```python
from build123d import *

# Parameters (mm, degrees)
EXTRUDE_THIN1_DEPTH = 3.175


with BuildPart() as part:
    # Sketch1 → Extrude-Thin1 (new, symmetric)
    with BuildSketch(Plane(origin=(0, 0, 0), x_dir=(0, 0, -1), z_dir=(1, 0, 0))):
        with BuildLine():
            ThreePointArc((-19.05, 0.3048), (-14.081230666, 0.814453346), (-9.525000281, 2.861201965))
            ThreePointArc((-9.525000281, 2.861201965), (0, 5.715), (9.525000281, 2.861201965))
            ThreePointArc((9.525000281, 2.861201965), (14.081230666, 0.814453346), (19.05, 0.3048))
            Line((19.05, 0.3048), (19.067602036, 0.000508679))
            ThreePointArc((19.067602036, 0.000508679), (14.002221921, 0.520071522), (9.357401999, 2.606616309))
            ThreePointArc((9.357401999, 2.606616309), (0, 5.4102), (-9.357401999, 2.606616309))
            ThreePointArc((-9.357401999, 2.606616309), (-14.002221921, 0.520071522), (-19.067602036, 0.000508679))
            Line((-19.067602036, 0.000508679), (-19.05, 0.3048))
        make_face()
    extrude(amount=EXTRUDE_THIN1_DEPTH, both=True)


solid = part.part
```
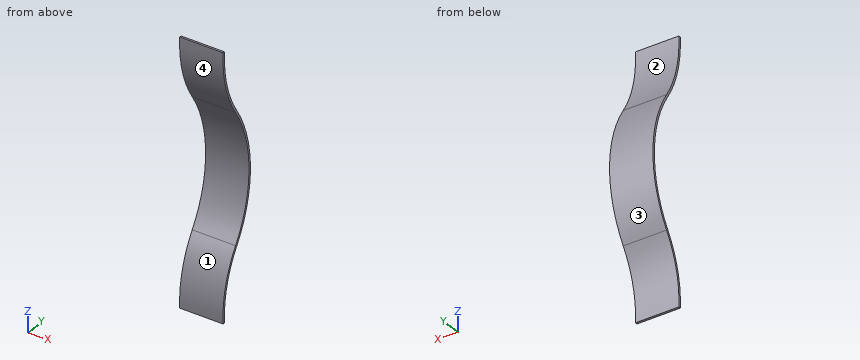
Part model, mm, in its own coordinate system. Face numbers are marked on the shaded views. A direction names the side the tool comes from. Coordinates: 2 decimals unless noted, no trailing zeros. Write each loop counter-clockwise with the first axis right and the second up, starting at its lowest first coordinate (ties: lowest second). Pieces come first, ordered by that corner, then holes.
Item 1: Pin check, flat tip, straight feed: pin 1 (1 mm diameter, centred on y = 2.5, z = 4, fed in from -X). Stop position of the tip, or through.
Item 2: Probe line 1 (Z direction, x = -1.25, y = 1.8); line 2 (Z direction, x = -0.25, y = 3.5); line 3 (Y direction, x = 1.5, z = 0) (3 decimals). List the from-to ranges inside material, lowest first.
Item 3: Slice it at C-C (y = 3.95). Write the cut outline in (x, z) (3 decimals), and give its area (3 significant figures).
Item 4: Which spindle directions (+Z, -Z, +X, -X, +Y, -Y) get a long thin tool onto all of the face, cutting with end or side? Do the marked faces 1 and 2. Say none if no direction does.
Item 5: Mould opens along Z. For the marked faces 3 and 4 say: released by +Z, released by -Z, zero draft, split by the parting line, or undercut.
Item 6: Slice it at D-D (z = -2). Write the cut outline in (x, y) (3 decimals).
Item 7: Slice it at A-A (y = 1.25). Write the cut outline in (x, z) (3 decimals).
Results found:
1. pin 1: passes through
2. line 1: z = -11.41 to -10.73, 10.73 to 11.41
2. line 2: z = -8.48 to -7.83, 7.83 to 8.48
2. line 3: y = 5.41 to 5.715
3. outline: (-3.175, -7.618) - (3.175, -7.618) - (3.175, -6.897) - (-3.175, -6.897) - close; (-3.175, 6.897) - (3.175, 6.897) - (3.175, 7.618) - (-3.175, 7.618) - close
3. area: 9.16 mm2
4. face 1: +X, -X, -Y
4. face 2: +X, -X, +Y
5. face 3: split by the parting line
5. face 4: undercut
6. outline: (-3.175, 5.292) - (3.175, 5.292) - (3.175, 5.599) - (-3.175, 5.599) - close
7. outline: (-3.175, -12.712) - (3.175, -12.712) - (3.175, -11.887) - (-3.175, -11.887) - close; (-3.175, 11.887) - (3.175, 11.887) - (3.175, 12.712) - (-3.175, 12.712) - close
